Model file for the job. Use its own axes, mm. A direction names the side the tool comes from. Give positions to 0.01 mm unless a question says otherwise; leave off trailing zeros. Loops run counter-clockwise (first coordinate to the right, second up) from the corner with the lowest first, then second, coordinate; pieces in that order, holes last. Notation, with made-up numbers: (-29, -8) - (27, -8) arc R20 cw to (27, 22) - close; hole circle Ø1 at (76.5, 15.25). An arc over 180 degrees is marked (long way). Use a Markdown table: item, result.
from build123d import *

# Parameters (mm, degrees)
PAD_DEPTH    = 4
PAD001_DEPTH = 4


with BuildPart() as part:
    # Sketch → Pad (new body)
    with BuildSketch(Plane.XZ):
        with BuildLine():
            Line((0, 0), (6.5, 0))
            Line((6.5, 0), (6.5, -40))
            Line((6.5, -40), (0, -40))
            Line((0, -40), (0, -27))
            ThreePointArc((0, -27), (1.202076, -26.502087), (1.7, -25.300015))
            Line((1.7, -18.700016), (1.7, -25.300015))
            ThreePointArc((1.7, -18.700016), (1.202087, -17.497924), (0, -17))
            Line((0, -17), (0, 0))
        make_face()
    pad = extrude(amount=-PAD_DEPTH)

    # Sketch001 → Pad001 (join)
    with BuildSketch(Plane.XY):
        with BuildLine():
            Line((0, 0), (6.5, 0))
            Line((6.5, 0), (6.5, 25))
            Line((6.5, 25), (0, 25))
            Line((0, 25), (0, 21))
            ThreePointArc((2.7, 18.3), (1.909188, 20.209188), (0, 21))
            Line((2.7, 11.7), (2.7, 18.3))
            ThreePointArc((0, 9), (1.909188, 9.790812), (2.7, 11.7))
            Line((0, 9), (0, 0))
        make_face()
    pad001 = extrude(amount=-PAD001_DEPTH)

    # Mirrored: Pad, Pad001 across Sketch V_Axis
    add(pad.mirror(Plane(origin=(0, 0, 0), x_dir=(0, -1, 0), z_dir=(1, 0, 0))))
    add(pad001.mirror(Plane(origin=(0, 0, 0), x_dir=(0, -1, 0), z_dir=(1, 0, 0))))


solid = part.part
(1) Pin check, flat tips, straight feed: P1, Ø6, axis at x = 1.5, z = -31.5, coming from the +Y side; P2, Ø1, axis at x = -4.5, y = 16, coming from the -Z side. Stop position of each tip, or through.
Computed:
| item | result |
|---|---|
| P1 | y = 4 |
| P2 | z = -4 |
(2) Slice it at C-C, the plane y = 13.5. Write the cut outline in (x, z), plus the area to 3 significant figures.
Computed:
| item | result |
|---|---|
| outline | (-6.5, -4) - (-2.7, -4) - (-2.7, 0) - (-6.5, 0) - close; (2.7, -4) - (6.5, -4) - (6.5, 0) - (2.7, 0) - close |
| area | 30.4 mm² |
(3) Drill centre lines: probe 1 along Y at (x, z) = (6.25, -14.5); probe 2 along Z at (x, y) = (-3, 19); probe 3 along Z at (x, y) = (0.25, 1.5). Where is each one in solid material? Low to high. Write a range as [from, to].
Computed:
| item | result |
|---|---|
| probe 1 | [0, 4] |
| probe 2 | [-4, 0] |
| probe 3 | [-40, -26.98], [-17.02, 0] |
(4) Slice it at B-B, the plane z = -21. Write the cut outline in (x, y).
Computed:
| item | result |
|---|---|
| outline | (-6.5, 0) - (-1.7, 0) - (-1.7, 4) - (-6.5, 4) - close; (1.7, 0) - (6.5, 0) - (6.5, 4) - (1.7, 4) - close |
(5) Slice it at A-A, the plane z = -3.5. Write the cut outline in (x, y).
Computed:
| item | result |
|---|---|
| outline | (-6.5, 0) - (6.5, 0) - (6.5, 25) - (-6.5, 25) - close; hole (-2.7, 11.7) arc R2.7 ccw to (0, 9) arc R2.7 ccw to (2.7, 11.7) - (2.7, 18.3) arc R2.7 ccw to (0, 21) arc R2.7 ccw to (-2.7, 18.3) - close |
(6) 3-axis set-ups, long thin cutter, end or side, ignore diameter. For faces 4 (the flat face through (6.5, 2, -12)), 5 (the flat face through (3, 15, -4)), 6 (the flat face through (2.7, 15, -2)), 7 (the flat face through (1.7, 2, -22)), 8 (the flat face through (3, 12, 0)): which of +Z, -Z, +X, -X, +Y, -Y reach the whole face in a straight line?
Computed:
| item | result |
|---|---|
| face 4 | +Z, -Z, +X, +Y, -Y |
| face 5 | -Z, +X, -X, +Y |
| face 6 | +Z, -Z |
| face 7 | +Y, -Y |
| face 8 | +Z, +X, -X, +Y, -Y |
(7) Slice it at D-D, the plane x = 1. Write the cut outline in (y, z).
Computed:
| item | result |
|---|---|
| outline | (0, -40) - (4, -40) - (4, -26.67) - (0, -26.67) - close; (0, -17.33) - (4, -17.33) - (4, -4) - (9.19, -4) - (9.19, 0) - (0, 0) - close; (20.81, -4) - (25, -4) - (25, 0) - (20.81, 0) - close |
(8) Mould opens along Z. For faces 1 (the flat face through (-1.7, 2, -22)), 2 (the flat face through (-3, 4, -22)), 3 (the flat face through (0, 2, -40)) say: pulls with the +Z half, pulls with the -Z half, needs draft (parallel to the pull), parting line crosses it, or undercut.
Computed:
| item | result |
|---|---|
| face 1 | undercut |
| face 2 | needs draft |
| face 3 | pulls with the -Z half |
